The figure shows three views and two pictorial views of one solid part (mm, origin at its lowest corner). Answer the questions. Coordinates: 2 decimals unless noted, no trailing zeros. Order: outer loops, then holes, each group sorted by start corner. A loop starts at its lowest first (then second) coordinate and runs counter-clockwise, first axis right, second up.
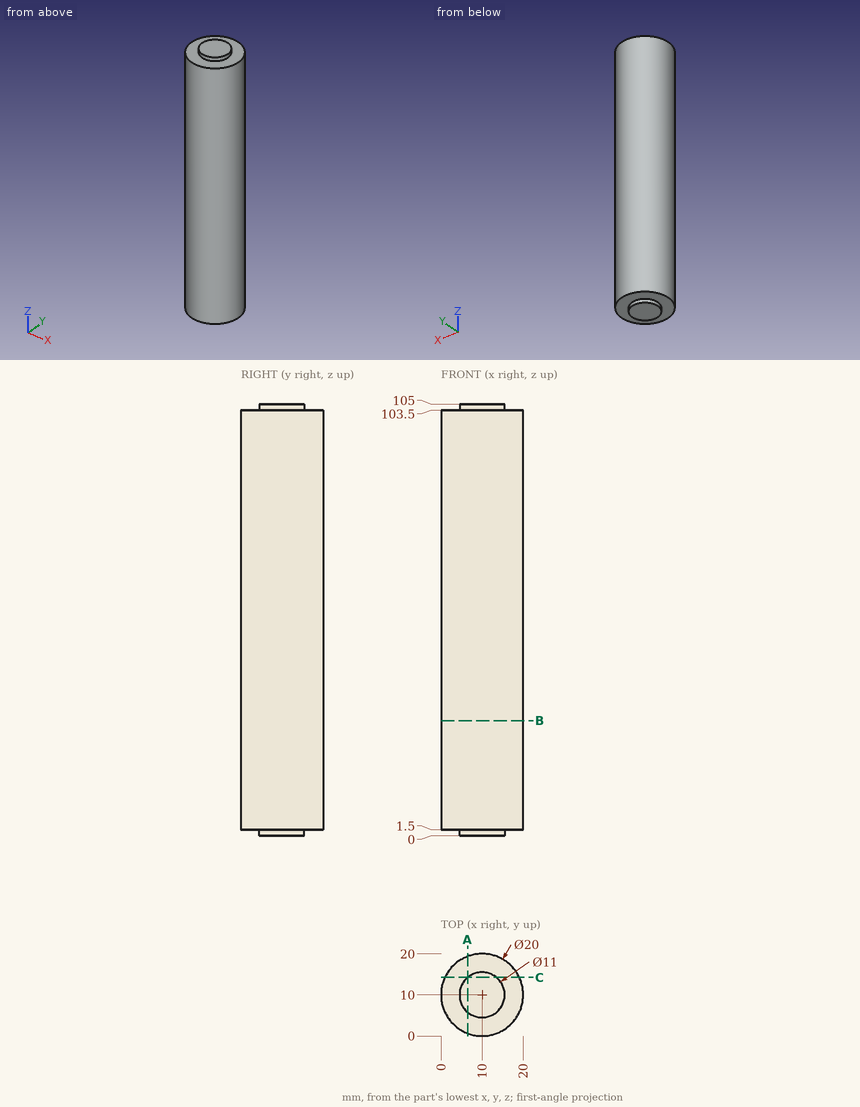
1) A cutting plane is placed at A-A, the plane x = 6.5. Write down the section's boundary in (y, z), plus the area to 3 significant figures.
2) Straight lines are drawn through the part: probe 1 along Y at (x, z) = (10.5, 29); probe 2 along Z at (x, y) = (3.75, 3); probe 3 along X at (y, z) = (3.25, 18). For each, find the intervals that lie inside material, in ascending order.
3) A cutting plane is placed at B-B, the plane z = 28. Write down the section's boundary in (x, y).
4) Each of these flat-tipped pins is pushed along its axis until it touches: P1, Ø4, axis at x = 15.5, z = 78, coming from the -Y side; P2, Ø6, axis at x = 14.5, z = 77.5, coming from the -Y side; P3, Ø5, axis at y = 15, z = 78.5, coming from the +X side. Where does it stop, or does it pass through?
5) A cutting plane is placed at C-C, the plane y = 14.25. Write down the section's boundary in (x, z).
Working result:
1. outline: (0.63, 1.5) - (5.76, 1.5) - (5.76, 0) - (14.24, 0) - (14.24, 1.5) - (19.37, 1.5) - (19.37, 103.5) - (14.24, 103.5) - (14.24, 105) - (5.76, 105) - (5.76, 103.5) - (0.63, 103.5) - close
1. area: 1,940 mm2
2. probe 1: y = 0.01 to 19.99
2. probe 2: z = 1.5 to 103.5
2. probe 3: x = 2.62 to 17.38
3. outline: circle Ø20 at (10, 10)
4. P1: stops at y = 0.63
4. P2: stops at y = 0.11
4. P3: stops at x = 19.68
5. outline: (0.95, 1.5) - (6.51, 1.5) - (6.51, 0) - (13.49, 0) - (13.49, 1.5) - (19.05, 1.5) - (19.05, 103.5) - (13.49, 103.5) - (13.49, 105) - (6.51, 105) - (6.51, 103.5) - (0.95, 103.5) - close
